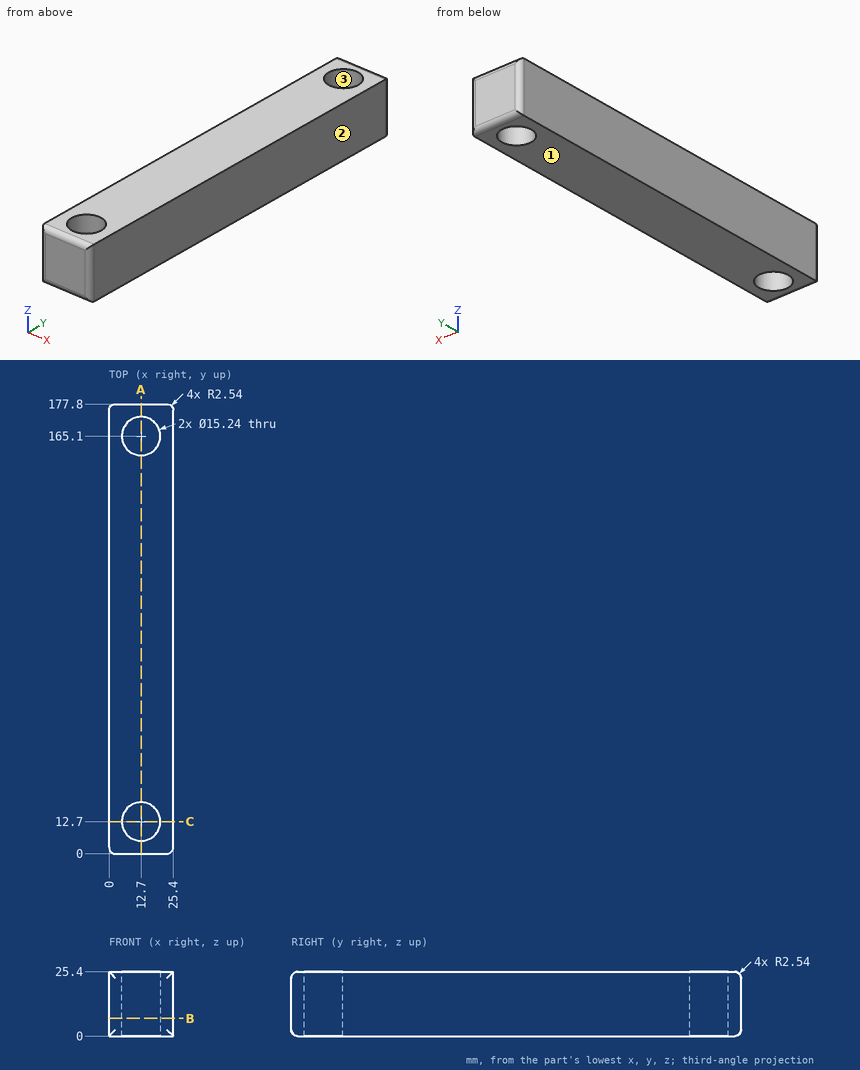
Geometry check sheet. Reference: drawing and pictorial views, mm from the part's lowest x, y, z. Give positions to 0.01 mm unless a question says otherwise; leave off trailing zeros. Write each loop counter-clockwise with the first axis right and the second up, starting at its lowest first coordinate (ties: lowest second). Pieces come first, ordered by that corner, then holes. Notation, with made-up numbers: (-26, 9.5) - (19, 9.5) arc R21 cw to (19, 33.5) - close; hole circle Ø6 at (59.5, -24.5). An arc over 180 degrees is marked (long way). Use a Markdown table: item, result.
Q1. Thickness scan on L1, parallel to Y at x = 12.7, z = 6.5; L2, parallel to Y at x = 19, z = 1; L3, parallel to X at y = 18, z = 16. Record the ranges inside material, lowest first. Write a range as [from, to].
Computed:
| item | result |
|---|---|
| L1 | y = [0, 5.08], [20.32, 157.48], [172.72, 177.8] |
| L2 | y = [0.52, 8.41], [16.99, 160.81], [169.39, 177.28] |
| L3 | x = [0, 7.23], [18.17, 25.4] |
Q2. Draft check along X on the marked faces 1, 2 and 3. Enter one of: pulls with the +X half, pulls with the -X half, needs draft (parallel to the pull), parting line crosses it, or undercut.
Computed:
| item | result |
|---|---|
| face 1 | needs draft |
| face 2 | pulls with the +X half |
| face 3 | undercut |
Q3. Section check A-A, the plane x = 12.7. Enter the section's corners in (y, z), then the cut area to 3 significant figures.
Computed:
| item | result |
|---|---|
| outline | (0, 2.54) arc R2.54 ccw to (2.54, 0) - (5.08, 0) - (5.08, 25.4) - (2.54, 25.4) arc R2.54 ccw to (0, 22.86) - close; (20.32, 0) - (157.48, 0) - (157.48, 25.4) - (20.32, 25.4) - close; (172.72, 0) - (175.26, 0) arc R2.54 ccw to (177.8, 2.54) - (177.8, 22.86) arc R2.54 ccw to (175.26, 25.4) - (172.72, 25.4) - close |
| area | 3,740 mm² |
Q4. Section check B-B, the plane z = 7. Enter the section's corners in (x, y), then the cut area to 3 significant figures.
Computed:
| item | result |
|---|---|
| outline | (0, 2.54) arc R2.54 ccw to (2.54, 0) - (22.86, 0) arc R2.54 ccw to (25.4, 2.54) - (25.4, 175.26) arc R2.54 ccw to (22.86, 177.8) - (2.54, 177.8) arc R2.54 ccw to (0, 175.26) - close; hole circle Ø15.24 at (12.7, 12.7); hole circle Ø15.24 at (12.7, 165.1) |
| area | 4,150 mm² |
Q5. Section check C-C, the plane y = 12.7. Enter the section's corners in (x, z).
Computed:
| item | result |
|---|---|
| outline | (0, 0) - (5.08, 0) - (5.08, 25.4) - (0, 25.4) - close; (20.32, 0) - (25.4, 0) - (25.4, 25.4) - (20.32, 25.4) - close |
